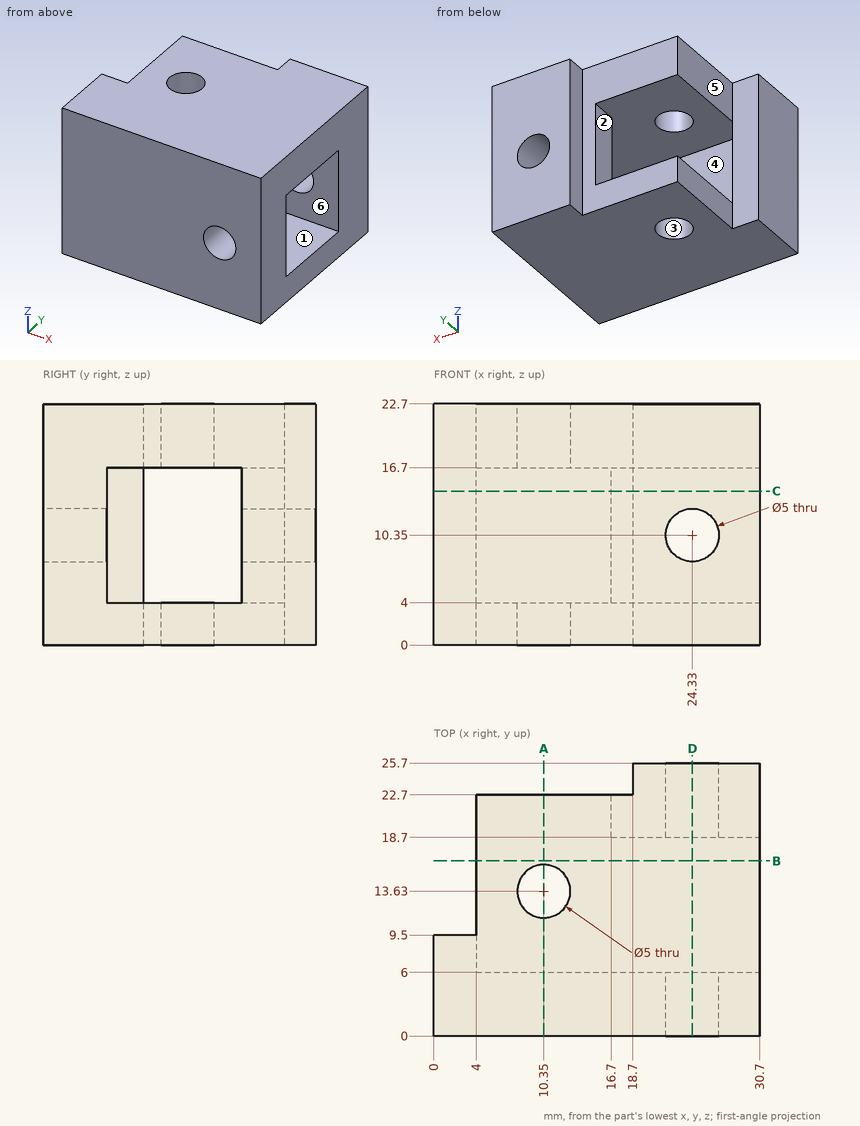
Design review of the part shown in the three views and the two pictorial views. Dimensions are in mm from the part's minimum x, y and z. A direction names the side the tool comes from. Round coordinates to 2 decimals unless told otherwise and drop trailing zeros. Write each loop counter-clockwise with the first axis right and the second up, starting at its lowest first coordinate (ties: lowest second). Pieces come first, ordered by that corner, then holes.
1) Take a section at A-A on x = 10.35. Give the boundary of the cut face in (y, z).
Answer below:
outline: (0, 0) - (11.13, 0) - (11.13, 4) - (6, 4) - (6, 16.7) - (11.13, 16.7) - (11.13, 22.7) - (0, 22.7) - close; (16.13, 0) - (22.7, 0) - (22.7, 4) - (16.13, 4) - close; (16.13, 16.7) - (22.7, 16.7) - (22.7, 22.7) - (16.13, 22.7) - close
2) Machinability: for the marked faces 4, 5 and 6, which of the approach directions +Z, -Z, +X, -X, +Y, -Y give a long, thin tool a straight path to every point of the face, cutting with its end or side? Answer none if there is none.
Answer below:
face 4: +X
face 5: +Z, -Z, -X, +Y
face 6: +X, -X
3) Insertion check: pin 1 Ø10 at (x, z) = (26, 7.5) entering from -Y; pin 2 Ø5 at (y, z) = (19.5, 21) entering from -X; pin 3 Ø12 at (x, z) = (11.5, 8) entering from +Y; pin 4 Ø2 at (y, z) = (20, 7.5) entering from -X. Each pin has a flat end and moves straight along its axis. Give the tip position at first contact, or say it passes through.
Answer below:
pin 1: stops at y = 0
pin 2: stops at x = 4
pin 3: stops at y = 22.7
pin 4: stops at x = 16.7
4) Take a section at B-B on y = 16.5. Give the boundary of the cut face in (x, z), then the cut area to 3 significant figures.
Answer below:
outline: (4, 0) - (30.7, 0) - (30.7, 4) - (4, 4) - close; (4, 16.7) - (30.7, 16.7) - (30.7, 22.7) - (4, 22.7) - close
area: 267 mm2
5) Take a section at D-D on x = 24.33. Give the boundary of the cut face in (y, z), then the cut area to 3 significant figures.
Answer below:
outline: (0, 0) - (25.7, 0) - (25.7, 7.85) - (18.7, 7.85) - (18.7, 4) - (6, 4) - (6, 7.85) - (0, 7.85) - close; (0, 12.85) - (6, 12.85) - (6, 16.7) - (18.7, 16.7) - (18.7, 12.85) - (25.7, 12.85) - (25.7, 22.7) - (0, 22.7) - close
area: 357 mm2
6) Take a section at C-C on z = 14.5. Give the boundary of the cut face in (x, y), then the cut area to 3 significant figures.
Answer below:
outline: (0, 0) - (30.7, 0) - (30.7, 6) - (4, 6) - (4, 9.5) - (0, 9.5) - close; (16.7, 18.7) - (30.7, 18.7) - (30.7, 25.7) - (18.7, 25.7) - (18.7, 22.7) - (16.7, 22.7) - close
area: 290 mm2
7) For line 1 along Y through (x, z) = (10.35, 1); line 2 along Z through (x, y) = (17, 15.5); line 3 along X through (y, z) = (19.25, 10.5), list the stretches that pass through material, from the lowest coordinate up.
Answer below:
line 1: y = 0 to 11.13, 16.13 to 22.7
line 2: z = 0 to 4, 16.7 to 22.7
line 3: x = 16.7 to 21.83, 26.83 to 30.7
8) Mouldability with a two-part tool opening along X and no side actions: class the marked faces 1, 2 and 3 as +X half, -X half, draft (parallel to the pull), parting line (faces both ways), or undercut.
Answer below:
face 1: draft
face 2: -X half
face 3: undercut
